Input: dimensioned drawing with shaded views. Units: mm. Origin: part minimum x, y, z. Round coordinates to 2 decimals unless told otherwise and drop trailing zeros. Loops run counter-clockwise (first coordinate to the right, second up) from the corner with the lowest first, then second, coordinate; pieces in that order, holes last.
Item 1: Ray query, L1, parallel to Z at x = 30, y = 0.6; L2, parallel to Z at x = 69.5, y = 2.75; L3, parallel to X at y = 0.1, z = 52.5. Return the intervals inside material, ascending.
Item 2: Section query C-C on x = 68.5. Return loops of the section in (y, z), then the cut area to 3 significant figures.
Item 3: Section query A-A on x = 33. Return loops of the section in (y, z), then the cut area to 3 significant figures.
Item 4: First-contact query: P1, Ø0.6, axis at y = 2, z = 51.5, coming from the -X side. Flat tip, straight axial feed; report the tip coordinate or a pass-through.
Item 5: Section query B-B on y = 1.8. Return loops of the section in (x, z).
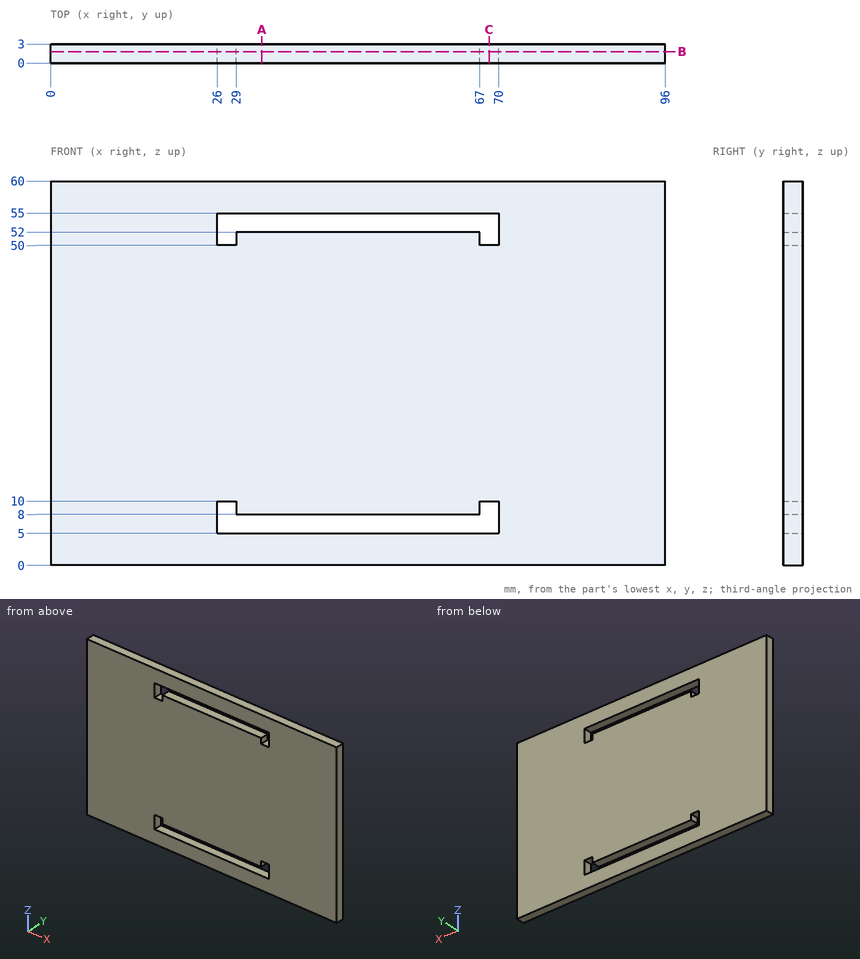
Data:
1. L1: z = 0 to 5, 8 to 52, 55 to 60
1. L2: z = 0 to 5, 10 to 50, 55 to 60
1. L3: x = 0 to 26, 70 to 96
2. outline: (0, 0) - (3, 0) - (3, 5) - (0, 5) - close; (0, 10) - (3, 10) - (3, 50) - (0, 50) - close; (0, 55) - (3, 55) - (3, 60) - (0, 60) - close
2. area: 150 mm2
3. outline: (0, 0) - (3, 0) - (3, 5) - (0, 5) - close; (0, 8) - (3, 8) - (3, 52) - (0, 52) - close; (0, 55) - (3, 55) - (3, 60) - (0, 60) - close
3. area: 162 mm2
4. P1: stops at x = 0
5. outline: (0, 0) - (96, 0) - (96, 60) - (0, 60) - close; hole (26, 5) - (70, 5) - (70, 10) - (67, 10) - (67, 8) - (29, 8) - (29, 10) - (26, 10) - close; hole (26, 50) - (29, 50) - (29, 52) - (67, 52) - (67, 50) - (70, 50) - (70, 55) - (26, 55) - close
